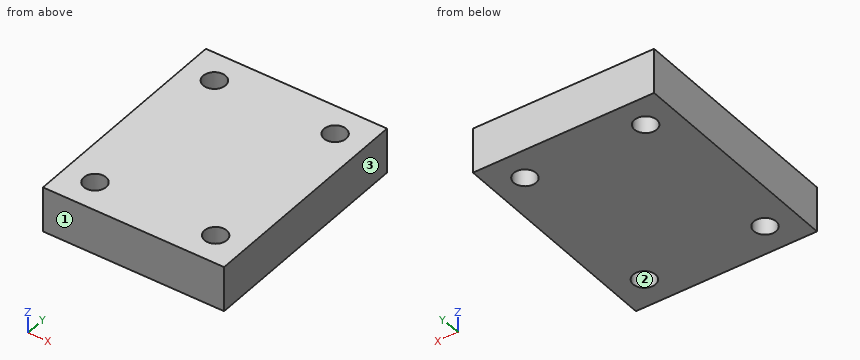
```python
from build123d import *

# Parameters (mm, degrees)
F0_W     = 95.25
F0_H     = 19.05
F1_DEPTH = 76.2
F2_R     = 4.699
F3_DEPTH = 25.4


with BuildPart() as f1:
    # F0 (on Right) → F1 (new body)
    with BuildSketch(Plane.YZ):
        with Locations((7.742904, -3.723968)):
            Rectangle(F0_W, F0_H)
    extrude(amount=F1_DEPTH)

    # F2 (on face) → F3 (cut)
    with BuildSketch(Plane.XY.offset(5.801032)):
        with Locations((63.5, -27.182096)):
            Circle(F2_R)
        with Locations((12.732774, -27.182096)):
            Circle(F2_R)
        with Locations((12.7, 42.667904)):
            Circle(F2_R)
        with Locations((63.5, 42.667904)):
            Circle(F2_R)
    extrude(amount=-F3_DEPTH, mode=Mode.SUBTRACT)


solid = f1.part
```
Geometry: final body of the model. Coordinates: model frame, mm. Face numbers are marked on the shaded views. Give positions to 0.01 mm unless a question says otherwise; leave off trailing zeros. Write each loop counter-clockwise with the first axis right and the second up, starting at its lowest first coordinate (ties: lowest second). Pieces come first, ordered by that corner, then holes.
1. Section query B-B, the plane y = -25. Return loops of the section in (x, z).
2. Draft query along Y for the marked faces 1, 2 and 3. Return one class per face: released by +Y, released by -Y, zero draft, split by the parting line, or undercut.
3. Section query C-C, the plane z = 1.5. Return loops of the section in (x, y), then the cut area to 3 significant figures.
4. Line query: probe 1 along Y at (x, z) = (12.7, -6.25); probe 2 along X at (y, z) = (-30, 0.5); probe 3 along Y at (x, z) = (62.5, -1). Output: solid intervals per line, ascending.
5. Section query A-A, the plane x = 63.5. Return loops of the section in (y, z).
Computed:
1. outline: (0, -13.25) - (8.57, -13.25) - (8.57, 5.8) - (0, 5.8) - close; (16.89, -13.25) - (59.34, -13.25) - (59.34, 5.8) - (16.89, 5.8) - close; (67.66, -13.25) - (76.2, -13.25) - (76.2, 5.8) - (67.66, 5.8) - close
2. face 1: released by -Y
2. face 2: undercut
2. face 3: zero draft
3. outline: (0, -39.88) - (76.2, -39.88) - (76.2, 55.37) - (0, 55.37) - close; hole circle Ø9.4 at (12.7, 42.67); hole circle Ø9.4 at (12.73, -27.18); hole circle Ø9.4 at (63.5, -27.18); hole circle Ø9.4 at (63.5, 42.67)
3. area: 6,980 mm2
4. probe 1: y = -39.88 to -31.88, -22.48 to 37.97, 47.37 to 55.37
4. probe 2: x = 0 to 8.97, 16.49 to 59.74, 67.26 to 76.2
4. probe 3: y = -39.88 to -31.77, -22.59 to 38.08, 47.26 to 55.37
5. outline: (-39.88, -13.25) - (-31.88, -13.25) - (-31.88, 5.8) - (-39.88, 5.8) - close; (-22.48, -13.25) - (37.97, -13.25) - (37.97, 5.8) - (-22.48, 5.8) - close; (47.37, -13.25) - (55.37, -13.25) - (55.37, 5.8) - (47.37, 5.8) - close
